```python
from build123d import *

# Parameters (mm, degrees)
F0_R      = 4.75
F1_DEPTH  = 0.5
F2_R      = 3.8
F3_DEPTH  = 1.3
F5_DEPTH  = 1.801
F6_R      = 3.15
F7_DEPTH  = 0.8
F8_R      = 2.165
F9_DEPTH  = 1.67
F10_R     = 3.14
F11_DEPTH = 0.67
F12_SIZE  = 0.5
F13_W     = 8.2
F13_H     = 8.2
F13_R     = 3.8
F14_DEPTH = 6
F15_SIZE  = 5.99999
F17_DEPTH = 6.001


# Not quite as in the source:
# - a fillet or chamfer is up to 0.001 mm smaller than in the source, because OpenCascade refuses the exact size


with BuildPart() as f1:
    # F0 (on Top) → F1 (new body)
    with BuildSketch(Plane.XY):
        Circle(F0_R)
    extrude(amount=F1_DEPTH)

    # F2 (on face) → F3 (join)
    with BuildSketch(Plane.XY.offset(0.5)):
        Circle(F2_R)
    extrude(amount=F3_DEPTH)

    # F4 (on face) → F5 (cut, through all)
    with BuildSketch(Plane(origin=(0, 0, 0), x_dir=(1, 0, 0), z_dir=(0, 0, -1))):
        with BuildLine():
            Line((-1.9965971051, 4.31), (0, 4.31))
            Line((0, 4.31), (1.9965971051, 4.31))
            ThreePointArc((1.9965971051, 4.31), (0, 4.75), (-1.9965971051, 4.31))
        make_face()
        with BuildLine():
            Line((0, -4.31), (-1.9965971051, -4.31))
            ThreePointArc((-1.9965971051, -4.31), (0, -4.75), (1.9965971051, -4.31))
            Line((1.9965971051, -4.31), (0, -4.31))
        make_face()
    extrude(amount=-F5_DEPTH, mode=Mode.SUBTRACT)

    # F6 (on face) → F7 (join)
    with BuildSketch(Plane(origin=(0, 0, 0), x_dir=(1, 0, 0), z_dir=(0, 0, -1))):
        Circle(F6_R)
    extrude(amount=F7_DEPTH)

    # F8 (on face) → F9 (join)
    with BuildSketch(Plane(origin=(0, 0, -0.8), x_dir=(1, 0, 0), z_dir=(0, 0, -1))):
        Circle(F8_R)
    extrude(amount=F9_DEPTH)

    # F10 (on face) → F11 (join)
    with BuildSketch(Plane(origin=(0, 0, -2.47), x_dir=(1, 0, 0), z_dir=(0, 0, -1))):
        Circle(F10_R)
    extrude(amount=F11_DEPTH)

    # F12
    f12_edges = [f1.edges().sort_by_distance(p)[0] for p in [
        (-3.14, 0, -3.14),
    ]]
    chamfer(f12_edges, length=F12_SIZE)

    # F13 (on face) → F14 (join)
    with BuildSketch(Plane.XY.offset(1.8)):
        Rectangle(F13_W, F13_H)
        Circle(F13_R, mode=Mode.SUBTRACT)
        Circle(F13_R)
    extrude(amount=F14_DEPTH)

    # F15 (size 6 in the source; OpenCascade refuses exactly that, so slightly less here)
    f15_edges = [f1.edges().sort_by_distance(p)[0] for p in [
        (0, 4.1, 7.8),
    ]]
    chamfer(f15_edges, length=F15_SIZE)

    # F16 (on face) → F17 (cut, through all)
    with BuildSketch(Plane(origin=(0, 0, 1.8), x_dir=(1, 0, 0), z_dir=(0, 0, -1))):
        with BuildLine():
            ThreePointArc((0, 4.1), (2.8991378029, 2.8991378029), (4.1, 0))
            Line((4.1, 0), (4.1, 4.1))
            Line((4.1, 4.1), (0, 4.1))
        make_face()
        with BuildLine():
            Line((4.1, -4.1), (4.1, 0))
            ThreePointArc((4.1, 0), (2.8991378029, -2.8991378029), (0, -4.1))
            Line((0, -4.1), (4.1, -4.1))
        make_face()
        with BuildLine():
            ThreePointArc((-4.1, 0), (-2.8991378029, 2.8991378029), (0, 4.1))
            Line((0, 4.1), (-4.1, 4.1))
            Line((-4.1, 4.1), (-4.1, 0))
        make_face()
        with BuildLine():
            Line((-4.1, -4.1), (0, -4.1))
            ThreePointArc((0, -4.1), (-2.8991378029, -2.8991378029), (-4.1, 0))
            Line((-4.1, 0), (-4.1, -4.1))
        make_face()
    extrude(amount=-F17_DEPTH, mode=Mode.SUBTRACT)


solid = f1.part
```
For this review, take the finished solid that the model builds, in its own axes (mm). A direction names the side the tool comes from. Coordinates: 2 decimals unless noted, no trailing zeros. Answer in a Markdown table with one row per item. Add a question column.
Q1. For probe 1 along Z at (x, y) = (-3.75, 2.75); probe 2 along Z at (x, y) = (1.75, 2.5); probe 3 along Y at (x, z) = (-0.25, 2), list the stretches that pass through material, from the lowest coordinate up.
Q2. Tool access review of faces 1 (the cylindrical face through (-3.796, 0.167, 1.141)), 2 (the flat face through (-0.1, 0.4, 5.5)), 3 (the cylindrical face through (-2.5, 1.917, -0.394)): name each direction out of +Z, -Z, +X, -X, +Y, -Y from which nothing blocks a thin tool from reaching the whole face with its end or side.
Q3. For P1, Ø4, axis at y = -2, z = 5, coming from the +X side; P2, Ø1.5, axis at y = -3.5, z = 4, coming from the -X side, all flat-tipped, find the tip position at first contact; note any pin that passes through.
Answer list:
| question | item | result |
|---|---|---|
| 1 | probe 1 | z = 0 to 0.5 |
| 1 | probe 2 | z = -2.73 to -2.47, -0.8 to 3.4 |
| 1 | probe 3 | y = -4.09 to 3.9 |
| 2 | face 1 | none |
| 2 | face 2 | +Z, +X, -X, +Y |
| 2 | face 3 | -Z |
| 3 | P1 | stops at x = 4.1 |
| 3 | P2 | stops at x = -3.04 |
